from build123d import *

# Parameters (mm, degrees)
EXTRUDE_1_DEPTH        = 450
SKETCH_2_R             = 3
SKETCH_2_R_2           = 1.75
CUT_EXTRUDE_1_DEPTH    = 4.5
SKETCH_2_2_R           = 1.75
CUT_EXTRUDE_2_DEPTH    = 9
PATTERN_LINEAR_1_COUNT = 18
PATTERN_LINEAR_1_PITCH = 25


with BuildPart() as part:
    # Эскиз1 → Бобышка-Вытянуть1 (new body)
    with BuildSketch(Plane.XY):
        with BuildLine():
            Line((-6, 3.7), (-5.7, 4))
            Line((-5.7, 4), (5.7, 4))
            Line((5.7, 4), (6, 3.7))
            Line((6, 3.7), (6, 2.451013544))
            ThreePointArc((6, 2.451013544), (5.597935912, 2.202976267), (5.354599002, 1.798050138))
            Line((5.354599002, 1.798050138), (4.643514056, 1.798050138))
            Line((4.643514056, 1.798050138), (4.643514056, 1.201949862))
            Line((4.643514056, 1.201949862), (5.354599002, 1.201949862))
            ThreePointArc((5.354599002, 1.201949862), (5.597935912, 0.797023733), (6, 0.548986456))
            Line((6, 0.548986456), (6, -3.7))
            Line((6, -3.7), (5.7, -4))
            Line((5.7, -4), (-5.7, -4))
            Line((-5.7, -4), (-6, -3.7))
            Line((-6, -3.7), (-6, 0.548986456))
            ThreePointArc((-6, 0.548986456), (-5.597935912, 0.797023733), (-5.354599002, 1.201949862))
            Line((-5.354599002, 1.201949862), (-4.643514056, 1.201949862))
            Line((-4.643514056, 1.201949862), (-4.643514056, 1.798050138))
            Line((-4.643514056, 1.798050138), (-5.354599002, 1.798050138))
            ThreePointArc((-5.354599002, 1.798050138), (-5.597935912, 2.202976267), (-6, 2.451013544))
            Line((-6, 2.451013544), (-6, 3.7))
        make_face()
    extrude(amount=EXTRUDE_1_DEPTH)

    # Эскиз2 → Вырез-Вытянуть1 (cut)
    with BuildSketch(Plane(origin=(0, 4, 0), x_dir=(1, 0, 0), z_dir=(0, 1, 0))):
        with Locations((0, -12.5)):
            Circle(SKETCH_2_R)
        with Locations((0, -12.5)):
            Circle(SKETCH_2_R_2, mode=Mode.SUBTRACT)
    cut_extrude_1 = extrude(amount=-CUT_EXTRUDE_1_DEPTH, mode=Mode.SUBTRACT)

    # Эскиз2<2> → Вырез-Вытянуть2 (cut, through all)
    with BuildSketch(Plane(origin=(0, 4, 0), x_dir=(1, 0, 0), z_dir=(0, 1, 0))):
        with Locations((0, -12.5)):
            Circle(SKETCH_2_2_R)
    cut_extrude_2 = extrude(amount=-CUT_EXTRUDE_2_DEPTH, mode=Mode.SUBTRACT)

    # Линейный массив1: Вырез-Вытянуть1, Вырез-Вытянуть2 ×18
    with Locations(*[(0, 0, i * PATTERN_LINEAR_1_PITCH) for i in range(1, PATTERN_LINEAR_1_COUNT)]):
        add(cut_extrude_1, mode=Mode.SUBTRACT)
        add(cut_extrude_2, mode=Mode.SUBTRACT)


solid = part.part
Could you check a few things on this model? Use its own coordinates, in mm. Give positions to 0.01 mm unless a question says otherwise; leave off trailing zeros. Order: outer loops, then holes, each group sorted by start corner. A loop starts at its lowest first (then second) coordinate and runs counter-clockwise, first axis right, second up. Notation, with made-up numbers: (61.5, 68) -> (103.5, 68) arc R31 ccw to (103.5, 103) -> close; hole circle Ø8 at (65, 32). An arc over 180 degrees is marked (long way). Answer in a Markdown table with one row per item. Add a question column.
Item 1: Please list where these lines run through material, in increasing order: probe 1 along X at (y, z) = (-3.5, 212); probe 2 along X at (y, z) = (1.55, 387.5); probe 3 along Y at (x, z) = (5, 103.5).
Item 2: Imagine slicing it at A-A (z = 53.5). List the corners of the cut face in (x, y) for me.
Item 3: I'm going to push flat-ended pins straight in: P1, Ø3, axis at x = 0, z = 437.5, coming from the -Y side; P2, Ø3, axis at x = -0.5, z = 387.5, coming from the +Y side. Where does each tip first touch, or does it pass through?
Result:
| question | item | result |
|---|---|---|
| 1 | probe 1 | -6 to -1.68, 1.68 to 6 |
| 1 | probe 2 | -4.64 to -3, 3 to 4.64 |
| 1 | probe 3 | -4 to 1.2, 1.8 to 4 |
| 2 | outline | (-6, -3.7) -> (-5.7, -4) -> (5.7, -4) -> (6, -3.7) -> (6, 0.55) arc R1 cw to (5.35, 1.2) -> (4.64, 1.2) -> (4.64, 1.8) -> (5.35, 1.8) arc R1 cw to (6, 2.45) -> (6, 3.7) -> (5.7, 4) -> (-5.7, 4) -> (-6, 3.7) -> (-6, 2.45) arc R1 cw to (-5.35, 1.8) -> (-4.64, 1.8) -> (-4.64, 1.2) -> (-5.35, 1.2) arc R1 cw to (-6, 0.55) -> close |
| 3 | P1 | through |
| 3 | P2 | y = -0.5 |
